Geometry: final body of the model. Coordinates: model frame, mm. A direction names the side the tool comes from. Coordinates: 2 decimals unless noted, no trailing zeros. Order: outer loops, then holes, each group sorted by start corner. A loop starts at its lowest first (then second) coordinate and runs counter-clockwise, first axis right, second up. Notation, with made-up numbers: (-10, -2.5) -> (2, -2.5) arc R30 cw to (2, 24.5) -> close; hole circle Ø4 at (84.25, 23.5). An arc over 180 degrees is marked (long way). Answer in a Markdown table with one row per item. Add a question column.
1) Section query B-B on y = 0. Return the cut outline in (x, z).
2) Contact query for flat-ended pins moving along their axis: P1, Ø0.5, axis at x = 2.5, z = 2, coming from the -Y side; P2, Ø3, axis at x = -2, z = 5, coming from the -Y side (3 decimals); P3, Ø4, axis at y = -1, z = 6, coming from the +X side; P4, Ø0.8, axis at y = 3, z = 7, coming from the +X side. Output: stop coordinate, or through.
3) Pull-direction query (Y, two-part tool) for faces 1 (the face through (-2.1, 0, 3.8)), 2 (the face through (0.06, 3.05, 0.62)), 3 (the face through (0, 2, 0)); classes: +Y half, -Y half, draft (parallel to the pull), parting line (faces both ways), or undercut.
4) Ray query, line 1 (Y direction, x = 0, z = 2.75); line 2 (X direction, y = 0, z = 7); line 3 (X direction, y = 3.5, z = 6). Return the intervals inside material, ascending. Write a range as from..to.
5) Section query A-A on x = 0. Return the cut outline in (y, z), then the cut area to 3 significant figures.
6) Set-up query: faces 4 (the face through (2, 0.8, 2)), 5 (the face through (2.725, -1.13, 2.873)), 6 (the face through (-0.819, 3, 8)), 7 (the face through (0, 3.729, 8)), 8 (the face through (0, -2.9, 7.8)). Return all of +Z, -Z, +X, -X, +Y, -Y with unobstructed straight access to the full face (end or side cutting, diameter ignored); none if empty.
7) Section query C-C on z = 1.5. Return the cut outline in (x, y), then the cut area to 3 significant figures.
8) Section query D-D on z = 5.75. Return the cut outline in (x, y).
```python
from build123d import *

# Parameters (mm, degrees)
SKETCH1_R               = 2.95
BOSS_EXTRUDE1_DEPTH     = 4.8
SKETCH10_R              = 3.05
BOSS_EXTRUDE2_DEPTH     = 1
CUT_EXTRUDE2_DEPTH      = 7.453293733
CUT_EXTRUDE2_DEPTH_BACK = 7.453293733
SKETCH1_4_R             = 1.45
CUT_EXTRUDE1_DEPTH      = 9
BOSS_EXTRUDE3_DEPTH     = 6
SKETCH12_R              = 1.45
CUT_EXTRUDE3_DEPTH      = 8.655520086
FILLET2_R               = 0.25


with BuildPart() as part:
    # Sketch1 → Boss-Extrude1 (new body)
    with BuildSketch(Plane(origin=(0, 0, 0), x_dir=(0, 1, 0), z_dir=(0, 0, 1))):
        with Locations(Location((0, 0, 0), (0, 0, 270))):
            Circle(SKETCH1_R)
    extrude(amount=BOSS_EXTRUDE1_DEPTH)

    # Sketch10 → Boss-Extrude2 (add)
    with BuildSketch(Plane(origin=(0, 0, 0), x_dir=(0, 1, 0), z_dir=(0, 0, 1))):
        with Locations(Location((0, 0, 0), (0, 0, 270))):
            Circle(SKETCH10_R)
    extrude(amount=BOSS_EXTRUDE2_DEPTH)

    # Sketch3 → Cut-Extrude2 (cut, two sides: drawn at the far end of the back side and taken through both)
    with BuildSketch(Plane.YZ.offset(-CUT_EXTRUDE2_DEPTH_BACK)):
        with BuildLine():
            Line((-0.8, -0.344662329), (-0.8, 3))
            ThreePointArc((-0.8, 3), (0, 3.8), (0.8, 3))
            Line((0.8, 3), (0.8, -0.344662329))
            ThreePointArc((0.8, -0.344662329), (0, -1.144662329), (-0.8, -0.344662329))
        make_face()
    extrude(amount=CUT_EXTRUDE2_DEPTH + CUT_EXTRUDE2_DEPTH_BACK, mode=Mode.SUBTRACT)

    # Sketch1<4> → Cut-Extrude1 (cut)
    with BuildSketch(Plane(origin=(0, 0, 0), x_dir=(0, 1, 0), z_dir=(0, 0, 1))):
        with Locations(Location((0, 0, 0), (0, 0, 56.514623377))):
            Circle(SKETCH1_4_R)
    extrude(amount=CUT_EXTRUDE1_DEPTH, mode=Mode.SUBTRACT)

    # Sketch11 → Boss-Extrude3 (add)
    with BuildSketch(Plane.XY.offset(4.8)):
        with BuildLine():
            Line((-0.818543418, 3.728872107), (0.981456582, 3.728872107))
            Line((0.981456582, 3.728872107), (0.981456582, 2.728872107))
            ThreePointArc((0.981456582, 2.728872107), (-0.085691473, -2.898733684), (-0.818543418, 2.782083153))
            Line((-0.818543418, 2.782083153), (-0.818543418, 3.728872107))
        make_face()
    extrude(amount=BOSS_EXTRUDE3_DEPTH)

    # Sketch12 → Cut-Extrude3 (cut, through all)
    with BuildSketch(Plane(origin=(0, 0, 4.8), x_dir=(1, 0, 0), z_dir=(0, 0, -1))):
        with Locations(Location((0, 0, 0), (0, 0, 180))):
            Circle(SKETCH12_R)
    extrude(amount=-CUT_EXTRUDE3_DEPTH, mode=Mode.SUBTRACT)

    # Fillet2
    fillet2_edges = [part.edges().sort_by_distance(p)[0] for p in [
        (0, 3.05, 0),
        (0, -3.05, 0),
        (2.076275596, 0.8, 0),
        (-2.076275596, -0.8, 0),
        (-2.076275596, 0.8, 0),
        (2.076275596, -0.8, 0),
        (0, 1.45, 0),
        (0, -1.45, 0),
    ]]
    fillet(fillet2_edges, radius=FILLET2_R)


solid = part.part
```
Result:
| question | item | result |
|---|---|---|
| 1 | outline | (-2.95, 3.8) -> (-1.45, 3.8) -> (-1.45, 10.8) -> (-2.9, 10.8) -> (-2.9, 4.8) -> (-2.95, 4.8) -> close; (1.45, 3.8) -> (2.95, 3.8) -> (2.95, 4.8) -> (2.9, 4.8) -> (2.9, 10.8) -> (1.45, 10.8) -> close |
| 2 | P1 | y = -1.91 |
| 2 | P2 | y = -2.905 |
| 2 | P3 | x = 2.95 |
| 2 | P4 | x = 1.28 |
| 3 | face 1 | undercut |
| 3 | face 2 | +Y half |
| 3 | face 3 | draft |
| 4 | line 1 | -2.95..-1.45, 1.45..2.95 |
| 4 | line 2 | -2.9..-1.45, 1.45..2.9 |
| 4 | line 3 | -0.82..0.98 |
| 5 | outline | (-3.05, 0.25) arc R0.25 ccw to (-2.8, 0) -> (-1.7, 0) arc R0.25 ccw to (-1.45, 0.25) -> (-1.45, 10.8) -> (-2.9, 10.8) -> (-2.9, 4.8) -> (-2.95, 4.8) -> (-2.95, 1) -> (-3.05, 1) -> close; (1.45, 0.25) arc R0.25 ccw to (1.7, 0) -> (2.8, 0) arc R0.25 ccw to (3.05, 0.25) -> (3.05, 1) -> (2.95, 1) -> (2.95, 4.8) -> (3.73, 4.8) -> (3.73, 10.8) -> (1.45, 10.8) -> close |
| 5 | area | 36.9 mm2 |
| 6 | face 4 | -Z, +X, -X |
| 6 | face 5 | none |
| 6 | face 6 | +Z, -X, +Y |
| 6 | face 7 | +Z, -Z, +X, -X, +Y |
| 6 | face 8 | +Z |
| 7 | outline | (-2.84, -0.8) arc R2.95 ccw to (2.84, -0.8) -> (1.21, -0.8) arc R1.45 cw to (-1.21, -0.8) -> close; (-2.84, 0.8) -> (-1.21, 0.8) arc R1.45 cw to (1.21, 0.8) -> (2.84, 0.8) arc R2.95 ccw to start |
| 7 | area | 15.8 mm2 |
| 8 | outline | (-0.82, 2.78) arc R2.9 ccw (long way) to (0.98, 2.73) -> (0.98, 3.73) -> (-0.82, 3.73) -> close; hole circle Ø2.9 at (0, 0) |
